Source: CAD feature listing. Evaluate the final solid. Frame: model axes, mm. A direction names the side the tool comes from. Coordinates: 2 decimals unless noted, no trailing zeros. Order: outer loops, then holes, each group sorted by start corner. A loop starts at its lowest first (then second) coordinate and runs counter-clockwise, first axis right, second up. Notation, with made-up numbers: (-25, -5) -> (-18, -5) arc R19 cw to (-18, 1) -> close; hole circle Ø10 at (3, 1). An arc over 180 degrees is marked (long way). Write each question's results on one line, items separated by ' | '. Start each with the question number.
from build123d import *

# Parameters (mm, degrees)
SKETCH1_W           = 44
SKETCH1_H           = 74
BOSS_EXTRUDE1_DEPTH = 1
SKETCH2_W           = 34
SKETCH2_H           = 12
CUT_EXTRUDE1_DEPTH  = 0.5
SKETCH3_W           = 6
SKETCH3_H           = 6
BOSS_EXTRUDE2_DEPTH = 1.5
SKETCH5_W           = 6.780779409
SKETCH5_H           = 6.387690747
BOSS_EXTRUDE5_DEPTH = 1.5
SKETCH7_W           = 6.4
SKETCH7_H           = 6.4
BOSS_EXTRUDE6_DEPTH = 1.5
SKETCH8_W           = 6.4
SKETCH8_H           = 6.4
BOSS_EXTRUDE7_DEPTH = 1.5
SKETCH9_W           = 6.4
SKETCH9_H           = 6.4
BOSS_EXTRUDE8_DEPTH = 1.5


with BuildPart() as part:
    # Sketch1 → Boss-Extrude1 (new body)
    with BuildSketch(Plane.XY):
        with Locations((22, 37)):
            Rectangle(SKETCH1_W, SKETCH1_H)
    extrude(amount=BOSS_EXTRUDE1_DEPTH)

    # Sketch2 → Cut-Extrude1 (cut)
    with BuildSketch(Plane.XY.offset(1)):
        with Locations((22, 50.703569151)):
            Rectangle(SKETCH2_W, SKETCH2_H)
    extrude(amount=-CUT_EXTRUDE1_DEPTH, mode=Mode.SUBTRACT)

    # Sketch3 → Boss-Extrude2 (add)
    with BuildSketch(Plane.XY.offset(1)):
        with Locations((22, 64.322360922)):
            Rectangle(SKETCH3_W, SKETCH3_H)
    extrude(amount=BOSS_EXTRUDE2_DEPTH)

    # Sketch5 → Boss-Extrude5 (add)
    with BuildSketch(Plane.XY.offset(1)):
        with Locations((8.782393761, 36.508639174)):
            Rectangle(SKETCH5_W, SKETCH5_H)
    extrude(amount=BOSS_EXTRUDE5_DEPTH)

    # Sketch7 → Boss-Extrude6 (add)
    with BuildSketch(Plane.XY.offset(1)):
        with Locations((9.083364884, 24.1147938)):
            Rectangle(SKETCH7_W, SKETCH7_H)
    extrude(amount=BOSS_EXTRUDE6_DEPTH)

    # Sketch8 → Boss-Extrude7 (add)
    with BuildSketch(Plane.XY.offset(1)):
        with Locations((9.279909214, 11.7147938)):
            Rectangle(SKETCH8_W, SKETCH8_H)
    extrude(amount=BOSS_EXTRUDE7_DEPTH)

    # Sketch9 → Boss-Extrude8 (add)
    with BuildSketch(Plane.XY.offset(1)):
        with Locations((35.1254887, 36.895573208)):
            Rectangle(SKETCH9_W, SKETCH9_H)
    extrude(amount=BOSS_EXTRUDE8_DEPTH)


solid = part.part
(1) First-contact query: P1, Ø0.8, axis at x = 7.5, z = 2, coming from the -Y side; P2, Ø9.5, axis at x = 28, y = 51.5, coming from the +Z side; P3, Ø0.8, axis at y = 37.5, z = 1.5, coming from the +X side. Flat tips, straight axial feed; report the tip coordinate or a pass-through.
(2) Section C-C on x = 8. Return the cut outline in (y, z), then the cut area to 3 significant figures.
(3) Draft query along X for faces 6 (the flat face through (22, 67.322, 2)), 7 (the flat face through (12.173, 36, 2)), 8 (the flat face through (19, 64, 2)). Return one class per face: released by +X, released by -X, zero draft, split by the parting line, or undercut.
(4) Section B-B on z = 1.8. Return the cut outline in (x, y).
(5) Reachability of faces 1 (the flat face through (25, 64, 2)), 2 (the flat face through (9, 33.315, 2)), 3 (the flat face through (22, 61.322, 2)), 4 (the flat face through (35, 33.696, 2)), 5 (the flat face through (35, 40.096, 2)) from +Z, -Z, +X, -X, +Y, -Y: full face, straight path, thin tool, end or side. Return the list, or none.
(6) Section D-D on y = 62.5. Return the cut outline in (x, z).
(7) Line query: L1, parallel to Y at x = 7.5, z = 1.8; L2, parallel to Y at x = 33.5, z = 0.95; L3, parallel to Z at x = 13.5, y = 27.5. Output: solid intervals per line, ascending.
(8) Section A-A on y = 47.5. Return the cut outline in (x, z), then the cut area to 3 significant figures.
Results list:
1) P1: stops at y = 8.51 | P2: stops at z = 0.5 | P3: stops at x = 38.33
2) outline: (0, 0) -> (74, 0) -> (74, 1) -> (56.7, 1) -> (56.7, 0.5) -> (44.7, 0.5) -> (44.7, 1) -> (39.7, 1) -> (39.7, 2.5) -> (33.31, 2.5) -> (33.31, 1) -> (27.31, 1) -> (27.31, 2.5) -> (20.91, 2.5) -> (20.91, 1) -> (14.91, 1) -> (14.91, 2.5) -> (8.51, 2.5) -> (8.51, 1) -> (0, 1) -> close | area: 96.8 mm²
3) face 6: zero draft | face 7: undercut | face 8: released by -X
4) outline: (5.39, 33.31) -> (12.17, 33.31) -> (12.17, 39.7) -> (5.39, 39.7) -> close; (5.88, 20.91) -> (12.28, 20.91) -> (12.28, 27.31) -> (5.88, 27.31) -> close; (6.08, 8.51) -> (12.48, 8.51) -> (12.48, 14.91) -> (6.08, 14.91) -> close; (19, 61.32) -> (25, 61.32) -> (25, 67.32) -> (19, 67.32) -> close; (31.93, 33.7) -> (38.33, 33.7) -> (38.33, 40.1) -> (31.93, 40.1) -> close
5) face 1: +Z, +X, +Y, -Y | face 2: +Z, +X, -X | face 3: +Z, +X, -X, -Y | face 4: +Z, +X, -Y | face 5: +Z, +X, -X, +Y
6) outline: (0, 0) -> (44, 0) -> (44, 1) -> (25, 1) -> (25, 2.5) -> (19, 2.5) -> (19, 1) -> (0, 1) -> close
7) L1: y = 8.51 to 14.91, 20.91 to 27.31, 33.31 to 39.7 | L2: y = 0 to 44.7, 56.7 to 74 | L3: z = 0 to 1
8) outline: (0, 0) -> (44, 0) -> (44, 1) -> (39, 1) -> (39, 0.5) -> (5, 0.5) -> (5, 1) -> (0, 1) -> close | area: 27.0 mm²
